Geometry check sheet. Reference: the model listing, model coordinates, mm. A direction names the side the tool comes from. Round coordinates to 2 decimals unless told otherwise and drop trailing zeros. Loops run counter-clockwise (first coordinate to the right, second up) from the corner with the lowest first, then second, coordinate; pieces in that order, holes last. Notation, with made-up numbers: M -30,-37 L -6,-37 A28 ccw -6,-10 Z; hole C 75.5,64 d1. An arc over 180 degrees is marked long. Use one line per item in the form item = value. Start each with the question number.
1. Cross-section at A-A (z = 63.5). Record the boundary of the cut face in (x, y), then the cut area to 3 significant figures.
2. Material ranges on line 1 (Z direction, x = 4.5, y = 3.25); line 2 (Z direction, x = 4.75, y = 4.5); line 3 (X direction, y = -0.5, z = 5), recorded low to high.
3. Go/stop test with flat-tipped pins: pin 1 (5 mm diameter, centred on x = 3, z = 93, fed in from -Y); pin 2 (2 mm diameter, centred on x = -4, y = -2.5, fed in from +Z). Record where each tip stops, or that it passes through.
4. Set-up check for faces 1 (the conical face through (3.386, 5.833, 0.065)), 2 (the flat face through (-1.37, 3.95, 5.3)): record each of +Z, -Z, +X, -X, +Y, -Y from which the full face is reachable in a straight line by a thin tool's end or side.
```python
from build123d import *

# Parameters (mm, degrees)
F1_DEPTH = 4.7
F4_R     = 5.8
F5_DEPTH = 0.6
F6_R     = 4
F7_DEPTH = 100
F8_SIZE  = 0.8


with BuildPart() as f1:
    # F0 (on Top) → F1 (new body)
    with BuildSketch(Plane.XY):
        Polygon((-3.7527767497, -6.5), (3.7527767497, -6.5), (7.5055534995, 0), (3.7527767497, 6.5), (-3.7527767497, 6.5), (-7.5055534995, 0), align=None)
    extrude(amount=F1_DEPTH)

    # F2 (on Front) → F3 (revolve, cut)
    with BuildSketch(Plane.XZ):
        Polygon((-7.5055534995, 0), (-6.5, 0), (-7.5055534995, 0.2694372481), align=None)
    revolve(axis=Axis((0, 0, 10.3672710247), (0, 0, 1)), mode=Mode.SUBTRACT)

    # F4 (on face) → F5 (join)
    with BuildSketch(Plane.XY.offset(4.7)):
        Circle(F4_R)
    extrude(amount=F5_DEPTH)

    # F6 (on face) → F7 (join)
    with BuildSketch(Plane.XY.offset(5.3)):
        Circle(F6_R)
    extrude(amount=F7_DEPTH)

    # F8
    f8_edges = [f1.edges().sort_by_distance(p)[0] for p in [
        (-4, 0, 105.3),
    ]]
    chamfer(f8_edges, length=F8_SIZE)


solid = f1.part
```
Reported:
q1.outline = C 0,0 d8
q1.area = 50.3 mm²
q2.line_1 = 0 to 5.3
q2.line_2 = 0.01 to 4.7
q2.line_3 = -5.78 to 5.78
q3.pin_1 = -3.97
q3.pin_2 = 104.78
q4.face_1 = -Z, +X, +Y
q4.face_2 = +Z
